Work out the finished part from the listing and answer in its coordinate system (mm). Face numbers are marked on the shaded views. A direction names the side the tool comes from. Round coordinates to 2 decimals unless told otherwise and drop trailing zeros. Order: outer loops, then holes, each group sorted by start corner. A loop starts at its lowest first (then second) coordinate and runs counter-clockwise, first axis right, second up. Notation, with made-up numbers: (-22.75, 6.25) - (-12.75, 6.25) arc R36 ccw to (-12.75, 42.25) - close; hole circle Ø7 at (9, 65). An arc over 180 degrees is marked (long way). Use one line per item in the form item = value. Start each with the question number.
Q1. The part is cut by section C-C on z = 6.25. Determine the outline of the cut face in (x, y).
Q2. Find the intervals of material crossed by line 1 (Y direction, x = 7.3, z = 3); line 2 (X direction, y = 5.25, z = 2); line 3 (X direction, y = 0, z = 4.75), in increasing order. Write a range as [from, to].
Q3. Given P1, Ø1.8, axis at y = -3, z = 4.5, coming from the -X side; P2, Ø2, axis at x = -0.5, z = 2, coming from the +Y side; P3, Ø1.5, axis at x = 5.5, z = 3, coming from the -Y side; P4, Ø1.5, axis at x = -7, y = 6.5, coming from the +Z side, each flat-ended and moving along its own axis, determine where each tip first touches the part or whether it passes through.
Q4. The part is cut by section B-B on y = -7.5. Determine the outline of the cut face in (x, z).
Q5. Which of the six approach directions +Z, -Z, +X, -X, +Y, -Y give full straight-line access (tool end or side, diameter ignored) to the marked faces 4, 5, 6 and 7?
Q6. The part is cut by section D-D on x = 3.25. Determine the outline of the cut face in (y, z), plus the area to 3 significant figures.
Q7. For a pull along Y with two mould halves and no side action, classify the marked faces 1, 2 and 3 as +Y half, -Y half, draft (parallel to the pull), parting line (faces both ways), or undercut.
Q8. The part is cut by section A-A on x = -7.5. Determine the outline of the cut face in (y, z).
from build123d import *

# Parameters (mm, degrees)
SKETCH_1_W                    = 21
SKETCH_1_H                    = 21
EXTRUDE_1_DEPTH               = 9.5
CUT_EXTRUDE_3_DEPTH           = 3.5
CUT_EXTRUDE_4_DEPTH           = 18.628102564
CHAMFER_1_SIZE                = 0.5
HOLE_WIZARD_2_561_D           = 1.778
HOLE_WIZARD_2_561_DEPTH       = 8.27
HOLE_WIZARD_2_561_CSINK_D     = 2.794
HOLE_WIZARD_2_561_CSINK_ANGLE = 110
HOLE_WIZARD_2_561_TIP         = 0.53416509


# Read off the part's stored shape, not the designer's step: Отверстие обработанное метчиком M31, Отверстие обработанное метчиком M32
with BuildPart() as part:
    # Эскиз1 → Бобышка-Вытянуть1 (new body)
    with BuildSketch(Plane.XY):
        Rectangle(SKETCH_1_W, SKETCH_1_H)
    extrude(amount=EXTRUDE_1_DEPTH)

    # Эскиз2 → Вырез-Вытянуть3 (cut)
    with BuildSketch(Plane.XY.offset(9.5)):
        with BuildLine():
            ThreePointArc((-4.5, -10.316653826), (4.385337165, -1.084119567), (-1.5, 10.297958971))
            Line((-1.5, 10.297958971), (-1.5, 10.5))
            Line((-1.5, 10.5), (-10.5, 10.5))
            Line((-10.5, 10.5), (-10.5, -10.5))
            Line((-10.5, -10.5), (-4.5, -10.5))
            Line((-4.5, -10.5), (-4.5, -10.316653826))
        make_face()
    extrude(amount=-CUT_EXTRUDE_3_DEPTH, mode=Mode.SUBTRACT)

    # Эскиз3 → Вырез-Вытянуть4 (cut, through all)
    with BuildSketch(Plane(origin=(0, 0, 0), x_dir=(-1, 0, 0), z_dir=(0, 0, -1))):
        Polygon((74.537024344, 6.5), (10.5, 6.5), (2.5, 6.5), (2.5, -6.5), (10.5, -6.5), (74.537024344, -6.5), (202.611073033, -6.5), (202.611073033, 6.5), align=None)
    extrude(amount=-CUT_EXTRUDE_4_DEPTH, mode=Mode.SUBTRACT)

    # Отверстие обработанное метчиком M31 outline → Отверстие обработанное метчиком M31 (revolve, cut)
    with BuildSketch(Plane(origin=(5.5, 0, 3), x_dir=(1, 0, 0), z_dir=(0, 0, 1))):
        Polygon((1.75, 10.5), (0, 10.5), (0, -10.5), (1.75, -10.5), (1.25, -10.149896231), (1.25, 10), align=None)
    revolve(axis=Axis((5.5, 0, 3), (0, 1, 0)), mode=Mode.SUBTRACT)

    # Hole Wizard M31 2 outline → Hole Wizard M31 2 (revolve, cut)
    with BuildSketch(Plane(origin=(-7.5, 0, 3), x_dir=(1, 0, 0), z_dir=(0, 0, 1))):
        Polygon((1.75, -6.5), (0, -6.5), (0, -10.5), (1.75, -10.5), (1.25, -10.149896231), (1.25, -7), align=None)
    revolve(axis=Axis((-7.5, 0, 3), (0, 1, 0)), mode=Mode.SUBTRACT)

    # Фаска1
    chamfer_1_edges = [part.edges().sort_by_distance(p)[0] for p in [
        (-10.5, -10.5, 3),
        (-10.5, 10.5, 3),
        (10.5, -10.5, 4.75),
        (10.5, 10.5, 4.75),
    ]]
    chamfer(chamfer_1_edges, length=CHAMFER_1_SIZE)

    # Отверстие обработанное метчиком #2-561
    with Locations(Plane(origin=(0, 10.5, 0), x_dir=(-1, 0, 0), z_dir=(0, 1, 0))):
        with Locations((0.5, 2)):
            CounterSinkHole(HOLE_WIZARD_2_561_D / 2, HOLE_WIZARD_2_561_CSINK_D / 2, depth=HOLE_WIZARD_2_561_DEPTH, counter_sink_angle=HOLE_WIZARD_2_561_CSINK_ANGLE)
            with Locations((0, 0, -(HOLE_WIZARD_2_561_DEPTH + HOLE_WIZARD_2_561_TIP / 2))):  # 118° drill point
                Cone(0, HOLE_WIZARD_2_561_D / 2, HOLE_WIZARD_2_561_TIP, mode=Mode.SUBTRACT)

    # Отверстие обработанное метчиком M32 outline → Отверстие обработанное метчиком M32 (revolve, cut)
    with BuildSketch(Plane(origin=(0, 5.5, 3), x_dir=(0, 1, 0), z_dir=(0, 0, -1))):
        Polygon((0, 5.5), (1.25, 5.5), (1.25, 10.149896231), (1.75, 10.5), (0, 10.5), align=None)
    revolve(axis=Axis((0, 5.5, 3), (1, 0, 0)), mode=Mode.SUBTRACT)


solid = part.part
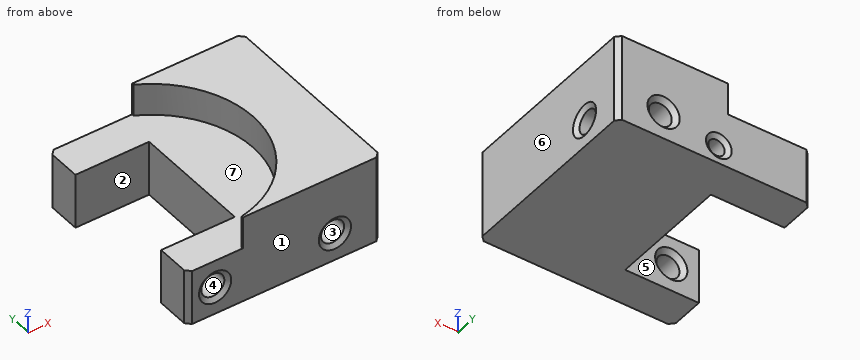
Found:
q1.outline = (-4.5, -10.5) - (10, -10.5) - (10.5, -10) - (10.5, 10) - (10, 10.5) - (-1.5, 10.5) - (-1.5, 10.3) arc R11 cw to (-4.5, -10.32) - close
q2.line_1 = [-10.5, 4.25], [6.75, 10.5]
q2.line_2 = [-2.5, -1.39], [0.39, 4.75]
q2.line_3 = [-2.5, 10.5]
q3.P1 = -2.5
q3.P2 = 10.22
q3.P3 = through
q3.P4 = 6
q4.outline = (-10.5, 0) - (10.5, 0) - (10.5, 9.5) - (1.05, 9.5) - (1.05, 6) - (-10.5, 6) - close; hole circle Ø2.5 at (-7.5, 3); hole circle Ø2.5 at (5.5, 3)
q5.face_4 = -Y
q5.face_5 = +Z, -Z, -X
q5.face_6 = +Z, -Z, +X, +Y, -Y
q5.face_7 = +Z, -X
q6.outline = (-10.5, 0) - (10.5, 0) - (10.5, 9.5) - (5.59, 9.5) - (5.59, 6) - (-4.59, 6) - (-4.59, 9.5) - (-10.5, 9.5) - close
q6.area = 164 mm²
q7.face_1 = -Y half
q7.face_2 = undercut
q7.face_3 = draft
q8.outline = (-10.5, 0) - (-6.5, 0) - (-6.5, 1.25) - (-7, 1.75) - (-10.15, 1.75) - (-10.5, 1.25) - close; (-10.5, 4.75) - (-10.15, 4.25) - (-7, 4.25) - (-6.5, 4.75) - (-6.5, 6) - (-10.5, 6) - close; (6.5, 0) - (10.5, 0) - (10.5, 6) - (6.5, 6) - close
